For this review, use the dimensioned drawing (mm, ordinates from the lowest corner) and the shaded views. A direction names the side the tool comes from. Coordinates: 2 decimals unless noted, no trailing zeros. Write each loop counter-clockwise with the first axis right and the second up, starting at its lowest first coordinate (ties: lowest second). Pieces come first, ordered by that corner, then holes.
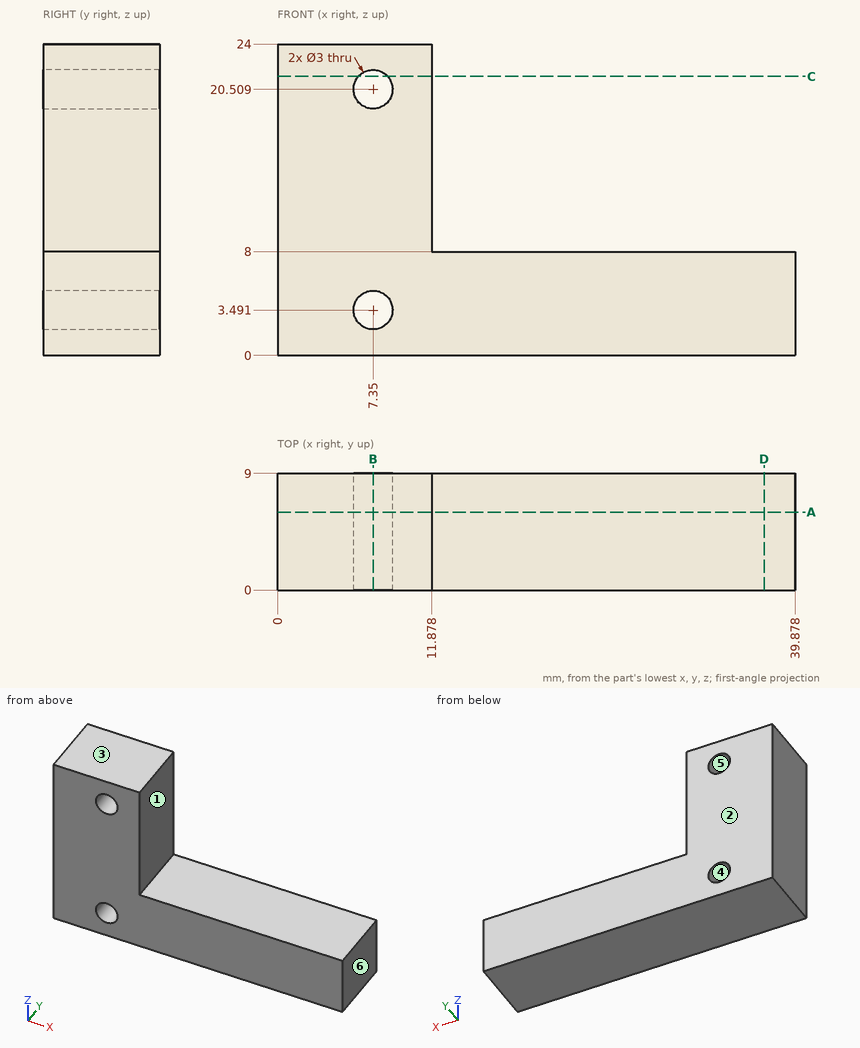
(1) Mouldability with a two-part tool opening along Z and no side actions: class the marked faces 3, 4, 5 and 6 as +Z half, -Z half, draft (parallel to the pull), parting line (faces both ways), or undercut.
(2) Insertion check: pin 1 Ø2.5 at (x, y) = (21.5, 3.5) entering from +Z; pin 2 Ø2.5 at (y, z) = (3, 13) entering from +X. Each pin has a flat end and moves straight along its axis. Give the tip position at first contact, or say it passes through.
(3) Wall thickness on line 1 (X direction, y = 1.25, z = 3.5); line 2 (X direction, y = 0.75, z = 15.75); line 3 (Z direction, x = 6, y = 5): over which ranges is each line inside the solid? List them lowest first.
(4) Consider section C-C (z = 21.5). Give the boundary of the cut face in (x, y), plus the area to 3 significant figures.
(5) Consider section D-D (x = 37.5). Give the boundary of the cut face in (y, z).
(6) Consider section A-A (y = 6). Give the boundary of the cut face in (x, z).
(7) Consider section B-B (x = 7.35). Give the boundary of the cut face in (y, z).
(8) For the marked faces 1 and 2, list the 3-axis set-ups (+Z, -Z, +X, -X, +Y, -Y) from which the entire face can be reached by the end or side of a thin tool; tool diameter is ignored.
Results:
1. face 3: +Z half
1. face 4: undercut
1. face 5: undercut
1. face 6: draft
2. pin 1: stops at z = 8
2. pin 2: stops at x = 11.88
3. line 1: x = 0 to 5.85, 8.85 to 39.88
3. line 2: x = 0 to 11.88
3. line 3: z = 0 to 2.84, 4.14 to 19.86, 21.16 to 24
4. outline: (0, 0) - (6.22, 0) - (6.22, 9) - (0, 9) - close; (8.48, 0) - (11.88, 0) - (11.88, 9) - (8.48, 9) - close
4. area: 86.6 mm2
5. outline: (0, 0) - (9, 0) - (9, 8) - (0, 8) - close
6. outline: (0, 0) - (39.88, 0) - (39.88, 8) - (11.88, 8) - (11.88, 24) - (0, 24) - close; hole circle Ø3 at (7.35, 3.49); hole circle Ø3 at (7.35, 20.51)
7. outline: (0, 0) - (9, 0) - (9, 1.99) - (0, 1.99) - close; (0, 4.99) - (9, 4.99) - (9, 19.01) - (0, 19.01) - close; (0, 22.01) - (9, 22.01) - (9, 24) - (0, 24) - close
8. face 1: +Z, +X, +Y, -Y
8. face 2: +Z, -Z, +X, -X, +Y
